Design review of the part built by this model. Coordinates are the model's own, in mm. Face numbers are marked on the shaded views. A direction names the side the tool comes from. Round coordinates to 2 decimals unless told otherwise and drop trailing zeros. Loops run counter-clockwise (first coordinate to the right, second up) from the corner with the lowest first, then second, coordinate; pieces in that order, holes last. Notation, with made-up numbers: (53.25, 5) -> (78.25, 5) arc R17 ccw to (78.25, 38) -> close; hole circle Ø4 at (38, 10.25). An arc over 180 degrees is marked (long way). Answer as CSV lines item,"result". Start each with the question number.
```python
from build123d import *

# Parameters (mm, degrees)
SKETCH1_W           = 50.8
SKETCH1_H           = 108.204
SKETCH1_R           = 4.1656
SKETCH1_H_2         = 19.05
BOSS_EXTRUDE1_DEPTH = 19.05
SKETCH1_3_W         = 50.8
SKETCH1_3_H         = 19.05
BOSS_EXTRUDE2_DEPTH = 110
SKETCH2_R           = 3.425
CUT_EXTRUDE1_DEPTH  = 176.710615832
FILLET1_R           = 2
SKETCH2_4_W         = 15
SKETCH2_4_H         = 25.4
BOSS_EXTRUDE3_DEPTH = 95
CHAMFER1_SIZE       = 15
CHAMFER1_SIZE2      = 46.165253058


with BuildPart() as part:
    # Sketch1 → Boss-Extrude1 (new body)
    # profile 1 of 2: a face of its own
    with BuildSketch(Plane.XY):
        with Locations((25.4, -54.102)):
            Rectangle(SKETCH1_W, SKETCH1_H)
        with Locations(Location((43.18, -100.076, 0), (0, 0, 180))):
            Circle(SKETCH1_R, mode=Mode.SUBTRACT)
        with Locations(Location((7.62, -100.076, 0), (0, 0, 180))):
            Circle(SKETCH1_R, mode=Mode.SUBTRACT)
        with Locations(Location((43.18, -8.128, 0), (0, 0, 180))):
            Circle(SKETCH1_R, mode=Mode.SUBTRACT)
        with Locations(Location((7.62, -8.128, 0), (0, 0, 180))):
            Circle(SKETCH1_R, mode=Mode.SUBTRACT)
    # profile 2 of 2: a face of its own
    with BuildSketch(Plane.XY):
        with Locations((25.4, 9.525)):
            Rectangle(SKETCH1_W, SKETCH1_H_2)
    extrude(amount=BOSS_EXTRUDE1_DEPTH)

    # Sketch1_3 → Boss-Extrude2 (add)
    with BuildSketch(Plane.XY):
        with Locations((25.4, 9.525)):
            Rectangle(SKETCH1_3_W, SKETCH1_3_H)
    extrude(amount=BOSS_EXTRUDE2_DEPTH)

    # Sketch2 → Cut-Extrude1 (cut, through all)
    with BuildSketch(Plane(origin=(0, 19.05, 0), x_dir=(1, 0, 0), z_dir=(0, 1, 0))):
        with Locations(Location((12.7, -59.15, 0), (0, 0, 270))):
            Circle(SKETCH2_R)
        with Locations(Location((12.7, -97.25, 0), (0, 0, 270))):
            Circle(SKETCH2_R)
        with Locations(Location((38.1, -97.25, 0), (0, 0, 270))):
            Circle(SKETCH2_R)
        with Locations(Location((38.1, -59.15, 0), (0, 0, 270))):
            Circle(SKETCH2_R)
    extrude(amount=-CUT_EXTRUDE1_DEPTH, mode=Mode.SUBTRACT)

    # Fillet1
    fillet1_edges = [part.edges().sort_by_distance(p)[0] for p in [
        (25.4, -108.204, 0),
        (25.4, 19.05, 0),
        (25.4, 0, 19.05),
        (25.4, 19.05, 110),
        (25.4, 0, 110),
        (25.4, -108.204, 19.05),
    ]]
    fillet(fillet1_edges, radius=FILLET1_R)

    # Sketch2_4 → Boss-Extrude3 (add)
    with BuildSketch(Plane(origin=(0, 19.05, 0), x_dir=(1, 0, 0), z_dir=(0, 1, 0))):
        with Locations((25.4, -31.75)):
            Rectangle(SKETCH2_4_W, SKETCH2_4_H)
    extrude(amount=-BOSS_EXTRUDE3_DEPTH)

    # Chamfer1
    chamfer1_edges = [part.edges().sort_by_distance(p)[0] for p in [
        (25.4, -75.95, 44.45),
    ]]
    chamfer1_side = [part.faces().sort_by_distance(p)[0] for p in [
        (25.4, -75.95, 31.75),
    ]]
    chamfer(chamfer1_edges, length=CHAMFER1_SIZE, length2=CHAMFER1_SIZE2, reference=chamfer1_side[0])


solid = part.part
```
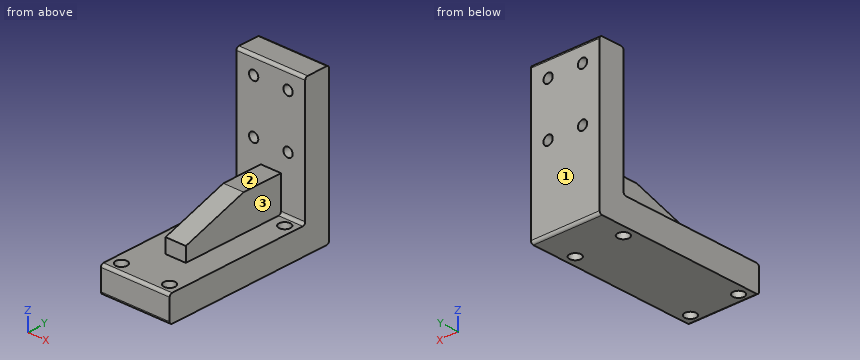
Q1. Add section C-C, the plane y = -24. Give the boundary of the cut face in (x, z).
Q2. To check wall thickness, follow probe 1 along X at (y, z) = (7.25, 97.25) (3 decimals); probe 2 along Y at (x, z) = (7.62, 5.5); probe 3 along Z at (x, y) = (12, 13). State the ranges of each line that lie inside material, in increasing order. Write a range as from..to.
Q3. Add section B-B, the plane x = 43.18. Give the boundary of the cut face in (y, z).
Q4. Machinability: for the marked faces 1, 2 and 3, which of the approach directions +Z, -Z, +X, -X, +Y, -Y give a long, thin tool a straight path to every point of the face, cutting with its end or side? Answer none if there is none.
Q5. Add section D-D, the plane x = 29. Give the boundary of the cut face in (y, z), and give its area (3 significant figures).
Q6. Add section A-A, the plane z = 59.15. Give the boundary of the cut face in (x, y) (3 decimals), and give its area (3 significant figures).
Q7. For pin 1 Ø12 at (x, y) = (29, -20) entering from +Z; pin 2 Ø6 at (x, z) = (30.5, 59) entering from -Y; pin 3 Ø3 at (x, z) = (27.5, 23) entering from -Y; pin 4 Ø7.5 at (x, y) = (7.62, -8.128) entering from +Z, all flat-tipped, find the tip position at first contact; note any pin that passes through.
Worked answers:
1,outline,"(0, 0) -> (50.8, 0) -> (50.8, 19.05) -> (32.9, 19.05) -> (32.9, 44.45) -> (17.9, 44.45) -> (17.9, 19.05) -> (0, 19.05) -> close"
2,probe 1,"x = 0..9.275, 16.125..34.675, 41.525..50.8"
2,probe 2,"y = -108.2..-104.24, -95.91..-12.29, -3.96..19.05"
2,probe 3,"z = 0..55.8, 62.5..93.9, 100.6..110"
3,outline,"(-108.2, 2) arc R2 ccw to (-106.2, 0) -> (-104.24, 0) -> (-104.24, 19.05) -> (-106.2, 19.05) arc R2 ccw to (-108.2, 17.05) -> close; (-95.91, 0) -> (-12.29, 0) -> (-12.29, 19.05) -> (-95.91, 19.05) -> close; (-3.96, 0) -> (17.05, 0) arc R2 ccw to (19.05, 2) -> (19.05, 108) arc R2 ccw to (17.05, 110) -> (2, 110) arc R2 ccw to (0, 108) -> (0, 21.05) arc R2 cw to (-2, 19.05) -> (-3.96, 19.05) -> close"
4,face 1,"+Z, -Z, +X, -X, +Y"
4,face 2,"+Z, +X, -X, -Y"
4,face 3,"+Z, +X, -Y"
5,outline,"(-108.2, 2) arc R2 ccw to (-106.2, 0) -> (17.05, 0) arc R2 ccw to (19.05, 2) -> (19.05, 108) arc R2 ccw to (17.05, 110) -> (2, 110) arc R2 ccw to (0, 108) -> (0, 44.45) -> (-29.78, 44.45) -> (-75.95, 29.45) -> (-75.95, 19.05) -> (-106.2, 19.05) arc R2 ccw to (-108.2, 17.05) -> close"
5,area,"5,740 mm^2"
6,outline,"(0, 0) -> (9.275, 0) -> (9.275, 19.05) -> (0, 19.05) -> close; (16.125, 0) -> (34.675, 0) -> (34.675, 19.05) -> (16.125, 19.05) -> close; (41.525, 0) -> (50.8, 0) -> (50.8, 19.05) -> (41.525, 19.05) -> close"
6,area,"707 mm^2"
7,pin 1,"stops at z = 44.45"
7,pin 2,"stops at y = 0"
7,pin 3,"stops at y = -75.95"
7,pin 4,"passes through"
